```python
from build123d import *

# Parameters (mm, degrees)
EXTRUDE_1_DEPTH           = 12
HOLE_WIZARD_1_D           = 9
HOLE_WIZARD_1_DEPTH       = 19.75
HOLE_WIZARD_1_CBORE_D     = 15
HOLE_WIZARD_1_CBORE_DEPTH = 9
HOLE_WIZARD_1_TIP         = 2.703872786
HOLE_WIZARD_2_D           = 9
HOLE_WIZARD_2_DEPTH       = 19.75
HOLE_WIZARD_2_CBORE_D     = 15
HOLE_WIZARD_2_CBORE_DEPTH = 9
HOLE_WIZARD_2_TIP         = 2.703872786


with BuildPart() as part:
    # 草图1 → 凸台-拉伸1 (new body)
    with BuildSketch(Plane.XY):
        with BuildLine():
            Line((-15, 12.5), (15, 12.5))
            ThreePointArc((15, 12.5), (27.5, 0), (15, -12.5))
            Line((15, -12.5), (-15, -12.5))
            ThreePointArc((-15, -12.5), (-27.5, 0), (-15, 12.5))
        make_face()
    extrude(amount=EXTRUDE_1_DEPTH)

    # 打孔尺寸(%根据)内六角圆柱头螺钉的类型1
    with Locations(Plane(origin=(0, 0, 0), x_dir=(-1, 0, 0), z_dir=(0, 0, -1))):
        with Locations((15, 0)):
            CounterBoreHole(HOLE_WIZARD_1_D / 2, HOLE_WIZARD_1_CBORE_D / 2, HOLE_WIZARD_1_CBORE_DEPTH, depth=HOLE_WIZARD_1_DEPTH)
            with Locations((0, 0, -(HOLE_WIZARD_1_DEPTH + HOLE_WIZARD_1_TIP / 2))):  # 118° drill point
                Cone(0, HOLE_WIZARD_1_D / 2, HOLE_WIZARD_1_TIP, mode=Mode.SUBTRACT)

    # 打孔尺寸(%根据)内六角圆柱头螺钉的类型2
    with Locations(Plane.XY.offset(12)):
        with Locations((15, 0)):
            CounterBoreHole(HOLE_WIZARD_2_D / 2, HOLE_WIZARD_2_CBORE_D / 2, HOLE_WIZARD_2_CBORE_DEPTH, depth=HOLE_WIZARD_2_DEPTH)
            with Locations((0, 0, -(HOLE_WIZARD_2_DEPTH + HOLE_WIZARD_2_TIP / 2))):  # 118° drill point
                Cone(0, HOLE_WIZARD_2_D / 2, HOLE_WIZARD_2_TIP, mode=Mode.SUBTRACT)


solid = part.part
```
CAD build for the part. Positions are in the model's coordinates, mm. A direction names the side the tool comes from. Coordinates: 2 decimals unless noted, no trailing zeros. Loops run counter-clockwise (first coordinate to the right, second up) from the corner with the lowest first, then second, coordinate; pieces in that order, holes last. Notation, with made-up numbers: (-33.5, 26.25) - (-26.5, 26.25) arc R29 ccw to (-26.5, 52.25) - close; hole circle Ø7 at (67.5, -18). An arc over 180 degrees is marked (long way). Use CSV: the item, a comma, the result in double quotes. Start each with the question number.
Q1. Drop flat-ended pins along their axis: P1, Ø13.5, axis at x = -15, y = 0, coming from the +Z side; P2, Ø11.5, axis at x = 15, y = 0, coming from the +Z side; P3, Ø1, axis at y = -5, z = 10, coming from the -X side; P4, Ø1.5, axis at y = 7, z = 9, coming from the -X side. Give the stop position or say it passes through.
Q2. Cut at A-A, the plane y = 0. List the corners of the cut face in (x, z).
Q3. Probe probe 1 along Y at (x, z) = (-15, 9.75); probe 2 along Y at (x, z) = (-15, 6.5); probe 3 along X at (y, z) = (3.5, 5.5). List the from-to ranges inside material, lowest first. Write a range as from..to.
Q4. Two-plate mould, pull along Y, no slides. Class faces 1 (the flat face through (0, 12.5, 6)), 2 (the flat face through (0, -12.5, 6)), 3 (the flat face through (20, 0, 3)): +Y half, -Y half, draft (parallel to the pull), parting line (faces both ways), or undercut.
Q5. Cut at C-C, the plane x = 14. List the corners of the cut face in (y, z).
Q6. Cut at D-D, the plane x = -11.5. List the corners of the cut face in (y, z), then the cut area to 3 significant figures.
Q7. 3-axis set-ups, long thin cutter, end or side, ignore diameter. For faces 4 (the cylindrical face through (27.497, 0.275, 5.916)), 5 (the cylindrical face through (-7.507, 0.33, 4.437)), 6 (the cylindrical face through (7.507, 0.33, 7.563)): which of +Z, -Z, +X, -X, +Y, -Y reach the whole face in a straight line?
Q8. Cut at B-B, the plane z = 6. List the corners of the cut face in (x, y), then the cut area to 3 significant figures.
Here are the results:
1,P1,"z = 12"
1,P2,"z = 3"
1,P3,"x = -26.66"
1,P4,"x = -25.83"
2,outline,"(-27.5, 0) - (-22.5, 0) - (-22.5, 9) - (-19.5, 9) - (-19.5, 12) - (-27.5, 12) - close; (-10.5, 9) - (-7.5, 9) - (-7.5, 0) - (10.5, 0) - (10.5, 3) - (7.5, 3) - (7.5, 12) - (-10.5, 12) - close; (19.5, 0) - (27.5, 0) - (27.5, 12) - (22.5, 12) - (22.5, 3) - (19.5, 3) - close"
3,probe 1,"-12.5..-4.5, 4.5..12.5"
3,probe 2,"-12.5..-7.5, 7.5..12.5"
3,probe 3,"-27..-21.63, -8.37..8.37, 21.63..27"
4,face 1,"+Y half"
4,face 2,"-Y half"
4,face 3,"undercut"
5,outline,"(-12.5, 0) - (-4.39, 0) - (-4.39, 3) - (-7.43, 3) - (-7.43, 12) - (-12.5, 12) - close; (4.39, 0) - (12.5, 0) - (12.5, 12) - (7.43, 12) - (7.43, 3) - (4.39, 3) - close"
6,outline,"(-12.5, 0) - (-6.63, 0) - (-6.63, 9) - (-2.83, 9) - (-2.83, 12) - (-12.5, 12) - close; (2.83, 9) - (6.63, 9) - (6.63, 0) - (12.5, 0) - (12.5, 12) - (2.83, 12) - close"
6,area,"164 mm2"
7,face 4,"+Z, -Z, +X"
7,face 5,"-Z"
7,face 6,"+Z"
8,outline,"(-15, -12.5) - (15, -12.5) arc R12.5 ccw to (15, 12.5) - (-15, 12.5) arc R12.5 ccw to start; hole circle Ø15 at (-15, 0); hole circle Ø15 at (15, 0)"
8,area,"887 mm2"
